Work out the finished part from the listing and answer in its coordinate system (mm). Coordinates: 2 decimals unless noted, no trailing zeros. Order: outer loops, then holes, each group sorted by start corner. A loop starts at its lowest first (then second) coordinate and runs counter-clockwise, first axis right, second up. Notation, with made-up numbers: M 12.25,-32.5 L 63.25,-32.5 A24 ccw 63.25,-8.5 Z; hole C 76,-23.5 d11. An arc over 180 degrees is marked long. Use a Markdown table: item, result. Add a question column.
from build123d import *

# Parameters (mm, degrees)
SKETCH1_W                                         = 88.9
SKETCH1_H                                         = 88.9
SKETCH1_R                                         = 4.191
SKETCH1_R_2                                       = 4.15
BOSS_EXTRUDE1_DEPTH                               = 6.35
CSK_FOR_5_16_FLAT_HEAD_MACHINE_SCREW1_D           = 8.4328
CSK_FOR_5_16_FLAT_HEAD_MACHINE_SCREW1_DEPTH       = 32.766
CSK_FOR_5_16_FLAT_HEAD_MACHINE_SCREW1_CSINK_D     = 16.129
CSK_FOR_5_16_FLAT_HEAD_MACHINE_SCREW1_CSINK_ANGLE = 82
CSK_FOR_5_16_FLAT_HEAD_MACHINE_SCREW1_TIP         = 2.533468714


with BuildPart() as part:
    # Sketch1 → Boss-Extrude1 (new body)
    with BuildSketch(Plane.XY):
        Rectangle(SKETCH1_W, SKETCH1_H)
        with Locations((-22.479, 0)):
            Circle(SKETCH1_R, mode=Mode.SUBTRACT)
        with Locations((22.521, 0)):
            Circle(SKETCH1_R_2, mode=Mode.SUBTRACT)
    extrude(amount=-BOSS_EXTRUDE1_DEPTH)

    # CSK for 5/16 Flat Head Machine Screw1
    with Locations(Plane(origin=(-22.479, 0, 0), x_dir=(1, 0, 0), z_dir=(0, 0, 1))):
        with Locations((0, 0), (45, 0)):
            CounterSinkHole(CSK_FOR_5_16_FLAT_HEAD_MACHINE_SCREW1_D / 2, CSK_FOR_5_16_FLAT_HEAD_MACHINE_SCREW1_CSINK_D / 2, depth=CSK_FOR_5_16_FLAT_HEAD_MACHINE_SCREW1_DEPTH, counter_sink_angle=CSK_FOR_5_16_FLAT_HEAD_MACHINE_SCREW1_CSINK_ANGLE)
            with Locations((0, 0, -(CSK_FOR_5_16_FLAT_HEAD_MACHINE_SCREW1_DEPTH + CSK_FOR_5_16_FLAT_HEAD_MACHINE_SCREW1_TIP / 2))):  # 118° drill point
                Cone(0, CSK_FOR_5_16_FLAT_HEAD_MACHINE_SCREW1_D / 2, CSK_FOR_5_16_FLAT_HEAD_MACHINE_SCREW1_TIP, mode=Mode.SUBTRACT)


solid = part.part
(1) A cutting plane is placed at B-B on z = -1. Write down the section's boundary in (x, y).
(2) A cutting plane is placed at A-A on y = 0. Write down the section's boundary in (x, z), plus the area to 3 significant figures.
(3) Given P1, Ø6, axis at x = 25.5, y = -2, coming from the +Z side; P2, Ø9.5, axis at x = -22.479, y = 0, coming from the +Z side, each flat-ended and moving along its own axis, determine where each tip first touches the part or whether it passes through.
(4) The mould has two halves that part along Y. Classify faces 1 (the cylindrical face through (26.733, 0.185, -5.402)), 2 (the cylindrical face through (-26.374, -1.615, -5.402)), 3 (the flat face through (-1, 1, -6.35)), 4 (the flat face through (-1, 44.45, -3)): pulls with the +Y half, pulls with the -Y half, needs draft (parallel to the pull), parting line crosses it, or undercut.
(5) Straight lines are drawn through the part: line 1 (X direction, y = 0, z = -4.9); line 2 (Y direction, x = 26, z = -2.75); line 3 (Y direction, x = 28, z = -2.25). For each, find the intervals that lie inside material, in ascending order.
From the geometry:
| question | item | result |
|---|---|---|
| 1 | outline | M -44.45,-44.45 L 44.45,-44.45 L 44.45,44.45 L -44.45,44.45 Z; hole C -22.48,0 d14.39; hole C 22.52,0 d14.39 |
| 2 | outline | M -44.45,-6.35 L -26.7,-6.35 L -26.7,-4.43 L -30.54,0 L -44.45,0 Z; M -18.26,-6.35 L 18.3,-6.35 L 18.3,-4.43 L 14.46,0 L -14.41,0 L -18.26,-4.43 Z; M 26.74,-6.35 L 44.45,-6.35 L 44.45,0 L 30.59,0 L 26.74,-4.43 Z |
| 2 | area | 423 mm2 |
| 3 | P1 | stops at z = -1.7 |
| 3 | P2 | stops at z = -3.81 |
| 4 | face 1 | undercut |
| 4 | face 2 | undercut |
| 4 | face 3 | needs draft |
| 4 | face 4 | pulls with the +Y half |
| 5 | line 1 | x = -44.45 to -26.7, -18.26 to 18.3, 26.74 to 44.45 |
| 5 | line 2 | y = -44.45 to -4.48, 4.48 to 44.45 |
| 5 | line 3 | y = -44.45 to -2.7, 2.7 to 44.45 |
